Can you work these out from the model? Positions are in its coordinate system, mm. Give positions to 0.01 mm unless a question says otherwise; leave off trailing zeros. Write each loop counter-clockwise with the first axis right and the second up, starting at its lowest first coordinate (ties: lowest second). Pieces come first, ordered by that corner, then holes. Notation, with made-up numbers: (34.25, 5) -> (80.25, 5) arc R20 cw to (80.25, 18) -> close; hole circle Ø6 at (18.5, 48.5). An arc over 180 degrees is marked (long way). One line per item, written item: value.
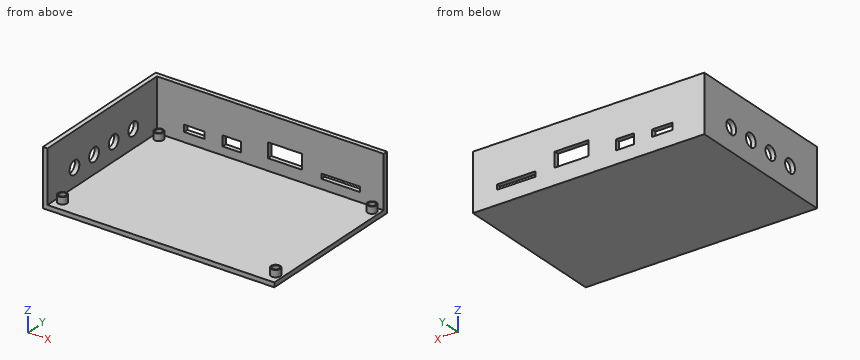
Autodesk Fusion 360 part; units mm, degrees
sketch "Sketch1" plane through (0, 0, 0) normal (0, 0, 1) x (1, 0, 0)
  line L0 (0, 0) -> (100, 0)
  line L1 (100, 0) -> (100, -65)
  line L2 (100, -65) -> (0, -65)
  line L3 (0, -65) -> (0, 0)
  dimension "d1" = 100
  dimension "d2" = 65
extrude "Extrude1" add sketch "Sketch1" along normal blind 2
sketch "Sketch2" plane through (0, 0, 2) normal (0, 0, 1) x (-1, 0, 0)
  line L0 (0, 65) -> (-100, 65)
  line L1 (-100, 65) -> (-100, 0)
  line L2 (-100, 0) -> (0, 0)
  line L3 (0, 0) -> (0, 65)
  line L4 (0, 65) -> (-120, 65)
  line L5 (-120, 65) -> (-210, 65)
  line L6 (-210, 65) -> (-290, 65)
  line L7 (-290, 65) -> (-370, 65)
  line L8 (-370, 65) -> (-490, 65)
  line L9 (-490, 65) -> (-640, 65)
  line L10 (-640, 65) -> (-725, 65)
  line L11 (-725, 65) -> (-895, 65)
  line L12 (-895, 65) -> (-1000, 65)
  line L13 (0, 0) -> (-1.5, 0)
  line L14 (-1.5, 0) -> (-1.5, 1.5)
  line L15 (-1.5, 1.5) -> (-1.5, 3)
  line L16 (-1.5, 3) -> (-3, 3)
  circle A0 centre (-3, 3) radius 1.5
  circle A1 centre (-3, 3) radius 2
  dimension "d5" = 120
  dimension "d6" = 90
  dimension "d7" = 80
  dimension "d8" = 80
  dimension "d9" = 120
  dimension "d10" = 150
  dimension "d11" = 85
  dimension "d12" = 170
  dimension "d13" = 105
  dimension "d14" = 1.5
  dimension "d15" = 1.5
  dimension "d16" = 1.5
  dimension "d17" = 1.5
  dimension "d18" = 3
extrude "Extrude2" add sketch "Sketch2" along normal blind 3 contours A1
pattern_linear "R-Pattern2" count 2 spacing 94 along (1, 0, 0) count 2 spacing 59 along (0, -1, 0) of "Extrude2"
sketch "Sketch4" plane through (0, 0, 0) normal (0, 0, -1) x (1, 0, 0)
  line L0 (100, 65) -> (0, 65)
  line L1 (0, 65) -> (0, 0)
  line L2 (0, 0) -> (100, 0)
  line L3 (100, 0) -> (100, 65)
  line L4 (0, 0) -> (-2, 0)
  line L5 (-2, 0) -> (-2, 65)
  line L6 (-2, 65) -> (0, 65)
  line L7 (0, 65) -> (0, 0)
  line L8 (-2, 65) -> (100, 65)
  line L9 (100, 65) -> (100, 67)
  line L10 (100, 67) -> (-2, 67)
  line L11 (-2, 67) -> (-2, 65)
  dimension "d37" = 2
  dimension "d38" = 2
extrude "Extrude6" add sketch "Sketch4" against normal blind 25 contours L0 L6 L8 L9 L10 L11 | L1 L4 L5 L6 L7 L8
sketch "Sketch5" plane through (0, -67, 0) normal (0, -1, 0) x (1, 0, 0)
  line L0 (-2, 0) -> (100, 0)
  line L1 (100, 0) -> (100, 25)
  line L2 (100, 25) -> (-2, 25)
  line L3 (-2, 25) -> (-2, 0)
  line L4 (0, 25) -> (0, 0) construction
  line L5 (0, 5) -> (100, 5) construction
  line L6 (0, 5) -> (100, 5)
  line L7 (100, 5) -> (100, 6.15)
  line L8 (100, 6.15) -> (0, 6.15)
  line L9 (0, 6.15) -> (0, 5)
  line L10 (0, 6.15) -> (12, 6.15)
  line L11 (12, 6.15) -> (21, 6.15)
  line L12 (21, 6.15) -> (21, 9.15)
  line L13 (21, 9.15) -> (12, 9.15)
  line L14 (12, 9.15) -> (12, 6.15)
  line L15 (21, 6.15) -> (29, 6.15)
  line L16 (29, 6.15) -> (37, 6.15)
  line L17 (37, 6.15) -> (37, 10.15)
  line L18 (37, 10.15) -> (29, 10.15)
  line L19 (29, 10.15) -> (29, 6.15)
  line L20 (37, 6.15) -> (49, 6.15)
  line L21 (49, 6.15) -> (64, 6.15)
  line L22 (64, 6.15) -> (64, 13.65)
  line L23 (64, 13.65) -> (49, 13.65)
  line L24 (49, 13.65) -> (49, 6.15)
  line L25 (64, 6.15) -> (72.5, 6.15)
  line L26 (72.5, 6.15) -> (89.5, 6.15)
  line L27 (89.5, 6.15) -> (89.5, 8.35)
  line L28 (89.5, 8.35) -> (72.5, 8.35)
  line L29 (72.5, 8.35) -> (72.5, 6.15)
  line L30 (89.5, 6.15) -> (100, 6.15)
  line L31 (49, 6.15) -> (49, 7.15)
  line L32 (49, 7.15) -> (64, 7.15)
  line L33 (29, 6.15) -> (29, 5.65)
  line L34 (29, 5.65) -> (37, 5.65)
  line L35 (37, 5.65) -> (37, 6.15)
  dimension "d41" = 1.15
  dimension "d42" = 12
  dimension "d43" = 9
  dimension "d44" = 3
  dimension "d45" = 8
  dimension "d46" = 8
  dimension "d47" = 4
  dimension "d48" = 12
  dimension "d49" = 15
  dimension "d50" = 7.5
  dimension "d51" = 8.5
  dimension "d52" = 17
  dimension "d53" = 2.2
  dimension "d73" = 1
  dimension "d74" = 0.5
extrude "Extrude7" cut sketch "Sketch5" against normal up to surface (2 mm away) contours L8 L26 L27 L28 L29 | L8 L11 L12 L13 L14 | L22 L23 L24 L32 | L8 L16 L17 L18 L19 | L8 L16 L33 L34 L35
sketch "Sketch6" plane through (-2, 0, 0) normal (-1, 0, 0) x (0, -1, 0)
  line L0 (0, 0) -> (67, 0)
  line L1 (67, 0) -> (67, 25)
  line L2 (67, 25) -> (0, 25)
  line L3 (0, 25) -> (0, 0)
  line L4 (65, 25) -> (65, 0)
  line L5 (67, 5) -> (0, 5)
  line L6 (67, 5) -> (0, 5)
  line L7 (0, 5) -> (0, 6.15)
  line L8 (0, 6.15) -> (67, 6.15) construction
  line L9 (67, 6.15) -> (67, 5)
  line L10 (65, 5) -> (65, 10)
  line L11 (65, 10) -> (0, 10)
  line L12 (65, 10) -> (50.5, 10)
  circle A0 centre (50.5, 10) radius 3
  line L13 (50.5, 10) -> (38.5, 10)
  circle A1 centre (38.5, 10) radius 3
  line L14 (38.5, 10) -> (26.5, 10)
  circle A2 centre (26.5, 10) radius 3
  line L15 (26.5, 10) -> (14.5, 10)
  circle A3 centre (14.5, 10) radius 3
  dimension "d56" = 67
  dimension "d57" = 1.15
  dimension "d58" = 5
  dimension "d59" = 14.5
  dimension "d60" = 6
  dimension "d61" = 12
  dimension "d62" = 12
  dimension "d63" = 12
ref_plane "WorkPlane1" through (50, -32.5, 13.5) normal (0, 1, 0) x (-1, 0, 0)
mirror "Mirror1" about plane through (50, -32.5, 13.5) normal (0, 1, 0) of "Extrude6"
extrude "Extrude8" cut sketch "Sketch6" against normal up to surface (2 mm away) contours L11 L12 A0 L13 | L11 L12 A0 L13 | L11 L15 A3 | L11 L15 A3 | L11 L13 A1 L14 | L11 L13 A1 L14 | L11 L14 A2 L15 | L11 L14 A2 L15
mirror "Mirror2" about plane through (50, -32.5, 13.5) normal (0, 1, 0) of "Extrude7"
sketch "Sketch7" plane through (0, 0, 25) normal (0, 0, 1) x (-1, 0, 0)
  line L0 (2, -2) -> (2, 67)
  line L1 (2, 67) -> (-100, 67)
  line L2 (-100, 67) -> (-100, 65)
  line L3 (-100, 65) -> (0, 65)
  line L4 (0, 65) -> (0, 0)
  line L5 (0, 0) -> (-100, 0)
  line L6 (-100, 0) -> (-100, -2)
  line L7 (-100, -2) -> (2, -2)
  line L8 (0, 65) -> (-100, 65)
  line L9 (-100, 65) -> (-100, 67)
  line L10 (-100, 67) -> (0, 67)
  line L11 (0, 67) -> (0, 65)
extrude "Extrude9" cut sketch "Sketch7" against normal blind 23 contours L1 L2 L3 L8 L9 L10 L11
1) If we section it at A-A (y = -26.5): Write out the boundary of the cut face in (x, z).
Answer list:
outline: (-2, 0) -> (100, 0) -> (100, 2) -> (0, 2) -> (0, 7) -> (-2, 7) -> close; (-2, 13) -> (0, 13) -> (0, 25) -> (-2, 25) -> close
2) I need wall thicknesses on L1, parallel to Y at x = 97, z = 3.05; L2, parallel to Y at x = -1.1, z = 10; L3, parallel to X at y = -62, z = 2.7. Which ranges of each line are inside material? Lowest first, please.
Answer list:
L1: y = -64 to -63.5, -60.5 to -60, -5 to -4.5, -1.5 to -1, 0 to 2
L2: y = -67 to -53.5, -47.5 to -41.5, -35.5 to -29.5, -23.5 to -17.5, -11.5 to 2
L3: x = -2 to 0, 1 to 1.5, 4.5 to 5, 95 to 95.5, 98.5 to 99
3) If we section it at B-B (x = 58): Write out the boundary of the cut face in (y, z).
Answer list:
outline: (-67, 0) -> (2, 0) -> (2, 7.15) -> (0, 7.15) -> (0, 2) -> (-67, 2) -> close; (0, 13.65) -> (2, 13.65) -> (2, 25) -> (0, 25) -> close
4) Will these pins go through, and if not, where does the flat tip stop? pin 1 (1 mm diameter, centred on x = 32, y = 1, fed in from -Z); pin 2 (4 mm diameter, centred on y = -27, z = 14.5, fed in from +X); pin 3 (1.5 mm diameter, centred on x = 2.5, y = -2.5, fed in from +Z); pin 4 (1.2 mm diameter, centred on x = 98, y = -3.5, fed in from +Z).
Answer list:
pin 1: stops at z = 0
pin 2: stops at x = 0
pin 3: stops at z = 2
pin 4: stops at z = 5
5) If we section it at D-D (z = 21.75): Write out the boundary of the cut face in (x, y), and give its area (3 significant figures).
Answer list:
outline: (-2, -67) -> (0, -67) -> (0, 0) -> (100, 0) -> (100, 2) -> (-2, 2) -> close
area: 338 mm^2
6) If we section it at C-C (x = 97): Write out the boundary of the cut face in (y, z).
Answer list:
outline: (-67, 0) -> (2, 0) -> (2, 25) -> (0, 25) -> (0, 2) -> (-1, 2) -> (-1, 5) -> (-1.5, 5) -> (-1.5, 2) -> (-4.5, 2) -> (-4.5, 5) -> (-5, 5) -> (-5, 2) -> (-60, 2) -> (-60, 5) -> (-60.5, 5) -> (-60.5, 2) -> (-63.5, 2) -> (-63.5, 5) -> (-64, 5) -> (-64, 2) -> (-67, 2) -> close
